The figure shows three views and two pictorial views of one solid part (mm, origin at its lowest corner). Answer the questions. Coordinates: 2 decimals unless noted, no trailing zeros. Write each loop counter-clockwise with the first axis right and the second up, starting at its lowest first coordinate (ties: lowest second). Pieces come first, ordered by that corner, then holes.
Item 1: Straight lines are drawn through the part: probe 1 along X at (y, z) = (7, 103); probe 2 along Z at (x, y) = (173, 4.5) (1 decimal); probe 3 along Z at (x, y) = (98, 16) (1 decimal). For each, find the intervals that lie inside material, in ascending order.
Item 2: Section B-B (x = 103.5) is taken. Give the vertices of the cut face in (y, z).
Item 3: Section D-D (x = 52.5) is taken. Give the vertices of the cut face in (y, z), then the cut area to 3 significant figures.
Item 4: Section A-A (z = 103.5) is taken. Give the vertices of the cut face in (x, y), then the cut area to 3 significant figures.
Item 5: Section C-C (z = 12.5) is taken. Give the vertices of the cut face in (x, y).
Item 6: Determine the mould class of the marked faces 1, 2 and 3 for opening direction X: released by +X, released by -X, zero draft, split by the parting line, or undercut.
Item 7: Each of these flat-tipped pins is pushed along its axis until it touches: P1, Ø8, axis at y = 14.5, z = 166.5, coming from the -X side; P2, Ø7, axis at x = 39.15, z = 39.15, coming from the +Y side; P3, Ø14, axis at x = 194.5, z = 103.5, coming from the +Y side; P4, Ø1.5, axis at x = 40, y = 3, coming from the +Z side. Where does it stop, or does it pass through?
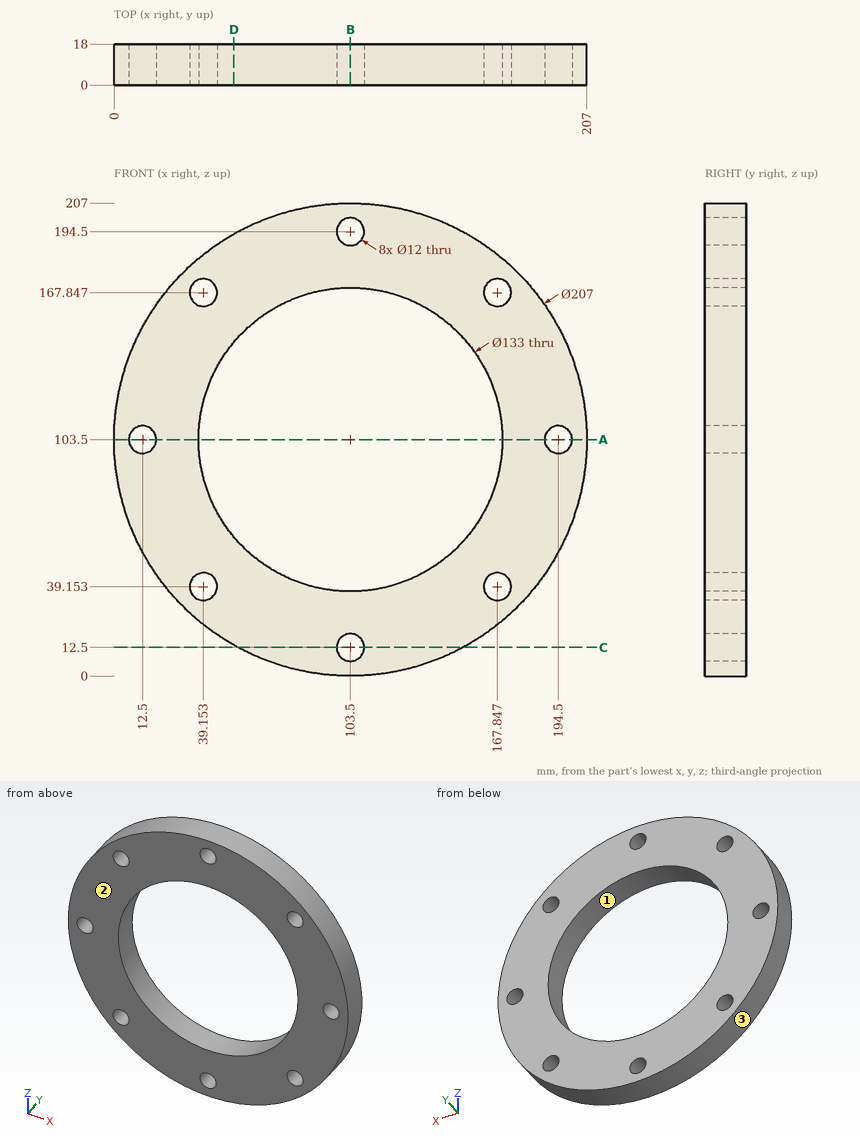
Established:
1. probe 1: x = 0 to 6.52, 18.48 to 37, 170 to 188.52, 200.48 to 207
1. probe 2: z = 26.8 to 36.1, 42.2 to 164.8, 170.9 to 180.2
1. probe 3: z = 0.1 to 10.1, 14.9 to 37.2, 169.8 to 192.1, 196.9 to 206.9
2. outline: (0, 0) - (18, 0) - (18, 6.5) - (0, 6.5) - close; (0, 18.5) - (18, 18.5) - (18, 37) - (0, 37) - close; (0, 170) - (18, 170) - (18, 188.5) - (0, 188.5) - close; (0, 200.5) - (18, 200.5) - (18, 207) - (0, 207) - close
3. outline: (0, 13.44) - (18, 13.44) - (18, 60.82) - (0, 60.82) - close; (0, 146.18) - (18, 146.18) - (18, 193.56) - (0, 193.56) - close
3. area: 1,710 mm2
4. outline: (0, 0) - (6.5, 0) - (6.5, 18) - (0, 18) - close; (18.5, 0) - (37, 0) - (37, 18) - (18.5, 18) - close; (170, 0) - (188.5, 0) - (188.5, 18) - (170, 18) - close; (200.5, 0) - (207, 0) - (207, 18) - (200.5, 18) - close
4. area: 900 mm2
5. outline: (54.19, 0) - (97.5, 0) - (97.5, 18) - (54.19, 18) - close; (109.5, 0) - (152.81, 0) - (152.81, 18) - (109.5, 18) - close
6. face 1: undercut
6. face 2: zero draft
6. face 3: split by the parting line
7. P1: stops at x = 18.46
7. P2: passes through
7. P3: stops at y = 18
7. P4: stops at z = 185.81
